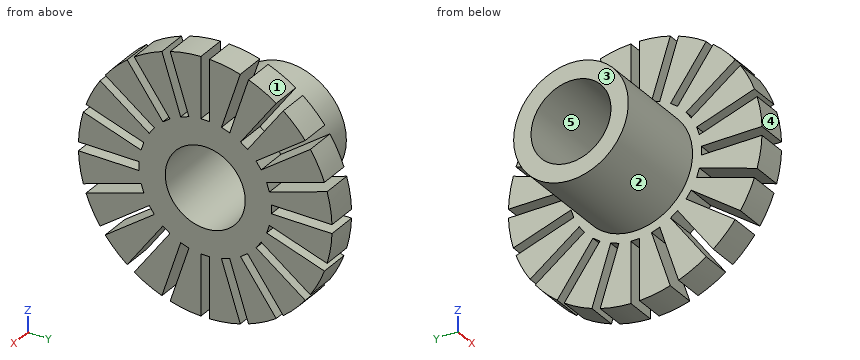
from build123d import *

# Parameters (mm, degrees)
POCKET_DEPTH       = 3.5
POLARPATTERN_COUNT = 20


with BuildPart() as part:
    # Sketch → Revolution (revolve)
    with BuildSketch(Plane.XY):
        Polygon((1.75, 4.6), (1.75, 14.6), (0, 14.6), (-1.75, 14.6), (-1.75, 6.6), (-13.25, 6.6), (-13.25, 4.6), align=None)
    revolve(axis=Axis((0, 0, 0), (1, 0, 0)))

    # Sketch001 (on Face4 of Revolution) → Pocket (cut)
    with BuildSketch(Plane(origin=(-1.75, 0, 0), x_dir=(0, -1, 0), z_dir=(-1, 0, 0))):
        Polygon((-0.5, 15.6), (0.5, 15.6), (0.5, 7.6), (0, 7.6), (-0.5, 7.6), align=None)
    pocket = extrude(amount=-POCKET_DEPTH, mode=Mode.SUBTRACT)

    # PolarPattern: Pocket ×20 about axis
    polarpattern_axis = Axis((-1.75, 0, 0), (-1, 0, 0))
    for i in range(1, POLARPATTERN_COUNT):
        add(pocket.rotate(polarpattern_axis, i * 360 / POLARPATTERN_COUNT), mode=Mode.SUBTRACT)


solid = part.part
Work out the finished part from the listing and answer in its coordinate system (mm). Face numbers are marked on the shaded views. A direction names the side the tool comes from. Give positions to 0.01 mm unless a question says otherwise; leave off trailing zeros. Loops run counter-clockwise (first coordinate to the right, second up) from the corner with the lowest first, then second, coordinate; pieces in that order, holes last. Notation, with made-up numbers: (65.25, -22.5) -> (119.25, -22.5) arc R21 ccw to (119.25, -0.5) -> close; hole circle Ø9 at (82, 66.5). An arc over 180 degrees is marked (long way). Use a Markdown table: item, result. Add a question column.
1. For the marked faces 1 and 2, determine the directions among +Z, -Z, +X, -X, +Y, -Y from which every point of the face is accessible in a straight line to the end or side of a thin tool.
2. Determine the mould class of the marked faces 3, 4 and 5 for opening direction Y: released by +Y, released by -Y, zero draft, split by the parting line, or undercut.
3. Flat-ended cylindrical pins translate along their axes: pin 1 Ø1.8 at (x, y) = (0.5, 12.5) entering from -Z; pin 2 Ø1.5 at (y, z) = (10, -5) entering from -X; pin 3 Ø0.8 at (x, z) = (-0.5, 0) entering from -Y. Find the tip coordinate at first contact, or state that the pin passes through.
4. Section C-C on x = -5.5 is taken. Determine the outline of the cut face in (y, z), and give its area (3 significant figures).
5. Section D-D on z = -12.5 is taken. Determine the outline of the cut face in (x, y).
6. Section A-A on y = 0 is taken. Determine the outline of the cut face in (x, z).
7. Find the intervals of material crossed by probe 1 along Z at (x, y) = (-7.25, 0); probe 2 along X at (y, z) = (8.25, -4); probe 3 along Z at (x, y) = (-1.5, 10.75), in increasing order.
Results below:
| question | item | result |
|---|---|---|
| 1 | face 1 | +Z, +X, -X, +Y |
| 1 | face 2 | -X |
| 2 | face 3 | zero draft |
| 2 | face 4 | released by -Y |
| 2 | face 5 | undercut |
| 3 | pin 1 | stops at z = -8.17 |
| 3 | pin 2 | stops at x = -1.75 |
| 3 | pin 3 | stops at y = -7.6 |
| 4 | outline | circle Ø13.2 at (0, 0); hole circle Ø9.2 at (0, 0) |
| 4 | area | 70.4 mm^2 |
| 5 | outline | (-1.75, -7.54) -> (1.75, -7.54) -> (1.75, -4.59) -> (-1.75, -4.59) -> close; (-1.75, -3.54) -> (1.75, -3.54) -> (1.75, -0.5) -> (-1.75, -0.5) -> close; (-1.75, 0.5) -> (1.75, 0.5) -> (1.75, 3.54) -> (-1.75, 3.54) -> close; (-1.75, 4.59) -> (1.75, 4.59) -> (1.75, 7.54) -> (-1.75, 7.54) -> close |
| 6 | outline | (-13.25, -6.6) -> (-1.75, -6.6) -> (-1.75, -7.6) -> (1.75, -7.6) -> (1.75, -4.6) -> (-13.25, -4.6) -> close; (-13.25, 4.6) -> (1.75, 4.6) -> (1.75, 7.6) -> (-1.75, 7.6) -> (-1.75, 6.6) -> (-13.25, 6.6) -> close |
| 7 | probe 1 | z = -6.6 to -4.6, 4.6 to 6.6 |
| 7 | probe 2 | x = -1.75 to 1.75 |
| 7 | probe 3 | z = -9.88 to -8.43, -7.19 to -4.02, -2.97 to -0.5, 0.5 to 2.97, 4.02 to 7.19, 8.43 to 9.88 |
